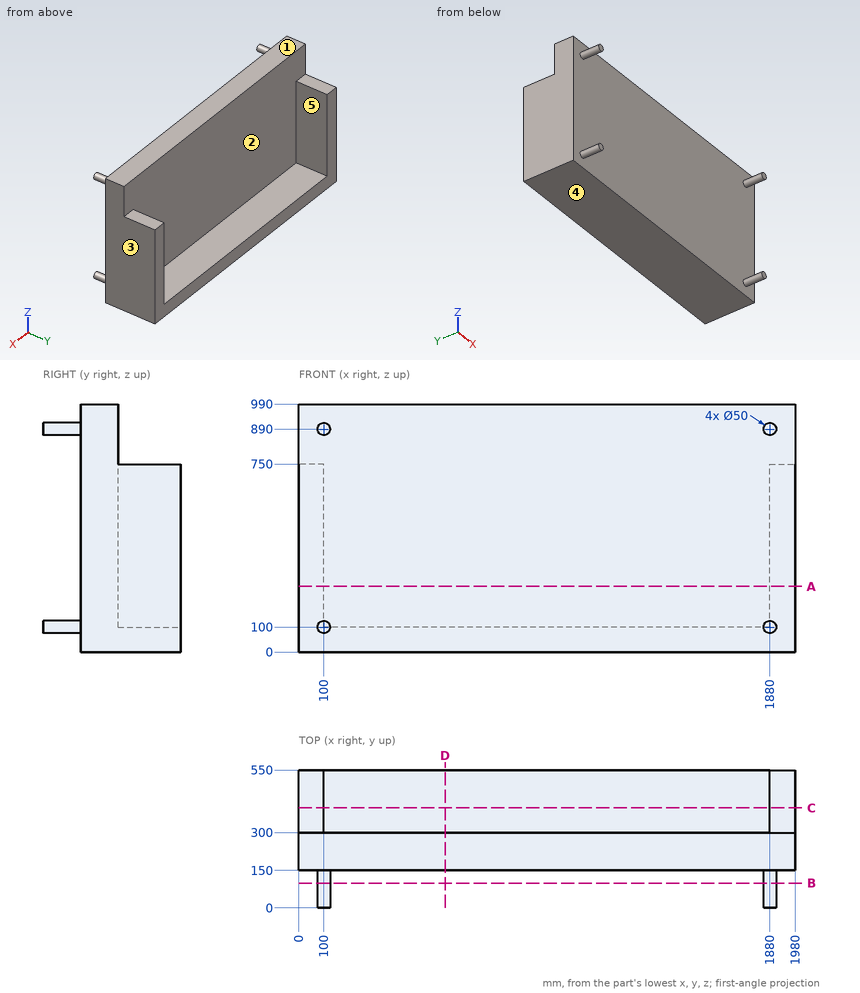
Could you check a few things on this drawing? It's one solid part, dimensions in mm from its lowest x, y, z. A direction names the side the tool comes from. Round coordinates to 2 decimals unless told otherwise and drop trailing zeros. Order: outer loops, then holes, each group sorted by start corner. A loop starts at its lowest first (then second) coordinate and runs counter-clockwise, first axis right, second up. Notation, with made-up numbers: M 11.5,14.5 L 25.5,14.5 A29 cw 25.5,37.5 Z; hole C -1,25 d3. An arc over 180 degrees is marked long. Return JSON: item names as keys, results as strings. Group by question number.
1. If we section it at A-A on z = 262.5: List the corners of the cut face in (x, y) for me.
2. If we section it at C-C on y = 399: List the corners of the cut face in (x, z) for me.
3. Please list where these lines run through material, in increasing order: probe 1 along X at (y, z) = (496, 588); probe 2 along Z at (x, y) = (314, 485.5); probe 3 along Y at (x, z) = (1884, 535.5).
4. If we section it at B-B on y = 99: List the corners of the cut face in (x, z) for me.
5. On a 3-axis mill with a long thin cutter (end or side, diameter ignored), from which of +Z, -Z, +X, -X, +Y, -Y can I reach the whole of each face in a straight line? I mean the marked faces 4 and 5. Say none if no direction works.
6. If we mould it in two halves opening along X, with no side actions, what happens to the marked faces 1, 2 and 3? For each: pulls with the +X half, pulls with the -X half, needs draft (parallel to the pull), parting line crosses it, or undercut.
7. I'm going to push flat-ended pins straight in: pin 1 Ø2 at (x, z) = (978, 394) entering from +Y; pin 2 Ø6 at (x, z) = (377, 366.5) entering from -Y. Where does each tip first touch, or does it pass through?
8. If we section it at D-D on x = 583.5: List the corners of the cut face in (y, z) for me, then the cut area to 4 significant figures.
Reply:
{
 "1": {"outline": "M 0,150 L 1980,150 L 1980,550 L 1880,550 L 1880,300 L 100,300 L 100,550 L 0,550 Z"},
 "2": {"outline": "M 0,0 L 1980,0 L 1980,750 L 1880,750 L 1880,100 L 100,100 L 100,750 L 0,750 Z"},
 "3": {"probe 1": "0 to 100, 1880 to 1980", "probe 2": "0 to 100", "probe 3": "150 to 550"},
 "4": {"outline": "C 100,100 d50; C 100,890 d50; C 1880,100 d50; C 1880,890 d50"},
 "5": {"face 4": "-Z, +X, -X, +Y, -Y", "face 5": "+Z, +Y"},
 "6": {"face 1": "needs draft", "face 2": "undercut", "face 3": "pulls with the +X half"},
 "7": {"pin 1": "y = 300", "pin 2": "y = 150"},
 "8": {"outline": "M 150,0 L 550,0 L 550,100 L 300,100 L 300,990 L 150,990 Z", "area": "173,500 mm^2"}
}
